```python
from build123d import *

# Parameters (mm, degrees)
SKETCH1_R           = 1.5
BOSS_EXTRUDE1_DEPTH = 10
FILLET1_R           = 1
FILLET2_R           = 1
FILLET3_R           = 1
FILLET4_R           = 1
FILLET5_R           = 1
FILLET6_R           = 1
FILLET7_R           = 1
FILLET8_R           = 1
SKETCH2_R           = 2.5
CUT_EXTRUDE1_DEPTH  = 10


with BuildPart() as part:
    # Sketch1 → Boss-Extrude1 (new body)
    with BuildSketch(Plane(origin=(0, 0, 0), x_dir=(1, 0, 0), z_dir=(0, 1, 0))):
        Polygon((37.3, 42.3), (5, 42.3), (0, 37.3), (0, 5), (5, 0), (37.3, 0), (42.3, 5), (42.3, 37.3), align=None)
        with Locations(Location((5, 5, 0), (0, 0, 270))):
            Circle(SKETCH1_R, mode=Mode.SUBTRACT)
        with Locations(Location((37.3, 5, 0), (0, 0, 270))):
            Circle(SKETCH1_R, mode=Mode.SUBTRACT)
        with Locations(Location((5, 37.3, 0), (0, 0, 270))):
            Circle(SKETCH1_R, mode=Mode.SUBTRACT)
        with Locations(Location((37.3, 37.3, 0), (0, 0, 270))):
            Circle(SKETCH1_R, mode=Mode.SUBTRACT)
    extrude(amount=BOSS_EXTRUDE1_DEPTH)

    # Fillet1
    fillet1_edges = [part.edges().sort_by_distance(p)[0] for p in [
        (0, 5, -5),
    ]]
    fillet(fillet1_edges, radius=FILLET1_R)

    # Fillet2
    fillet2_edges = [part.edges().sort_by_distance(p)[0] for p in [
        (5, 5, 0),
    ]]
    fillet(fillet2_edges, radius=FILLET2_R)

    # Fillet3
    fillet3_edges = [part.edges().sort_by_distance(p)[0] for p in [
        (37.3, 5, 0),
    ]]
    fillet(fillet3_edges, radius=FILLET3_R)

    # Fillet4
    fillet4_edges = [part.edges().sort_by_distance(p)[0] for p in [
        (42.3, 5, -5),
    ]]
    fillet(fillet4_edges, radius=FILLET4_R)

    # Fillet5
    fillet5_edges = [part.edges().sort_by_distance(p)[0] for p in [
        (42.3, 5, -37.3),
    ]]
    fillet(fillet5_edges, radius=FILLET5_R)

    # Fillet6
    fillet6_edges = [part.edges().sort_by_distance(p)[0] for p in [
        (37.3, 5, -42.3),
    ]]
    fillet(fillet6_edges, radius=FILLET6_R)

    # Fillet7
    fillet7_edges = [part.edges().sort_by_distance(p)[0] for p in [
        (5, 5, -42.3),
    ]]
    fillet(fillet7_edges, radius=FILLET7_R)

    # Fillet8
    fillet8_edges = [part.edges().sort_by_distance(p)[0] for p in [
        (0, 5, -37.3),
    ]]
    fillet(fillet8_edges, radius=FILLET8_R)

    # Sketch2 → Cut-Extrude1 (cut)
    with BuildSketch(Plane(origin=(0, 10, 0), x_dir=(1, 0, 0), z_dir=(0, 1, 0))):
        with Locations(Location((21.15, 21.15, 0), (0, 0, 270))):
            Circle(SKETCH2_R)
    extrude(amount=-CUT_EXTRUDE1_DEPTH, mode=Mode.SUBTRACT)


solid = part.part
```
Build history of the part. All positions in model axes, mm. Give positions to 0.01 mm unless a question says otherwise; leave off trailing zeros. Order: outer loops, then holes, each group sorted by start corner. A loop starts at its lowest first (then second) coordinate and runs counter-clockwise, first axis right, second up. Notation, with made-up numbers: M 26,88.25 L 60,88.25 A28 cw 60,115.25 Z; hole C 11,-21.75 d8. An arc over 180 degrees is marked long. Write item = value, one per line. Start each with the question number.
(1) Slice it at C-C on y = 1.75. Write the cut outline in (x, z), plus the area to 3 significant figures.
(2) Slice it at B-B on x = 21.15. Write the cut outline in (y, z), plus the area to 3 significant figures.
(3) Slice it at A-A on z = -21.15. Write the cut outline in (x, y), plus the area to 3 significant figures.
(4) Slice it at D-D on z = -3. Write the cut outline in (x, y).
(5) Pin check, flat tip, straight feed: pin 1 Ø2.5 at (x, z) = (5, -5) entering from -Y. Stop position of the tip, or through.
(6) Two-plate mould, pull along Z, no slides. Class faces 1 (the flat face through (26, 0, -21)), 2 (the cylindrical face through (5.07, 4.93, -6.5)), 3 (the flat face through (21, 5, -42.3)): released by +Z, released by -Z, zero draft, split by the parting line, or undercut.
(7) Probe L1, parallel to X at y = 6, z = -5; L2, parallel to X at y = 2.75, z = -5.5; L3, parallel to Z at x = 22.5, y = 1.5. List the from-to ranges inside material, lowest first. Write a range as [from, to].
Responses:
q1.outline = M 0,-36.89 A1 ccw 0.29,-37.59 L 4.71,-42.01 A1 ccw 5.41,-42.3 L 36.89,-42.3 A1 ccw 37.59,-42.01 L 42.01,-37.59 A1 ccw 42.3,-36.89 L 42.3,-5.41 A1 ccw 42.01,-4.71 L 37.59,-0.29 A1 ccw 36.89,0 L 5.41,0 A1 ccw 4.71,-0.29 L 0.29,-4.71 A1 ccw 0,-5.41 Z; hole C 5,-37.3 d3; hole C 5,-5 d3; hole C 21.15,-21.15 d5; hole C 37.3,-37.3 d3; hole C 37.3,-5 d3
q1.area = 1,690 mm2
q2.outline = M 0,-42.3 L 10,-42.3 L 10,-23.65 L 0,-23.65 Z; M 0,-18.65 L 10,-18.65 L 10,0 L 0,0 Z
q2.area = 373 mm2
q3.outline = M 0,0 L 18.65,0 L 18.65,10 L 0,10 Z; M 23.65,0 L 42.3,0 L 42.3,10 L 23.65,10 Z
q3.area = 373 mm2
q4.outline = M 2,0 L 40.3,0 L 40.3,10 L 2,10 Z
q5.pin_1 = through
q6.face_1 = zero draft
q6.face_2 = undercut
q6.face_3 = released by -Z
q7.L1 = [0.09, 3.5], [6.5, 35.8], [38.8, 42.21]
q7.L2 = [0, 3.59], [6.41, 35.89], [38.71, 42.3]
q7.L3 = [-42.3, -23.25], [-19.05, 0]
